```python
from build123d import *

# Parameters (mm, degrees)
SKETCH1_W                    = 80
SKETCH1_H                    = 40
SKETCH1_R                    = 10
BOSS_EXTRUDE1_DEPTH          = 3
SKETCH2_W                    = 80
SKETCH2_H                    = 4.5
BOSS_EXTRUDE2_DEPTH          = 8
SKETCH3_W                    = 2.5
SKETCH3_H                    = 6
CUT_EXTRUDE1_DEPTH           = 80
SKETCH5_R                    = 1.75
CUT_EXTRUDE3_DEPTH           = 1
SKETCH4_R                    = 3.75
CUT_EXTRUDE4_DEPTH           = 2
CUT_EXTRUDE4_DRAFT           = -45
CUT_EXTRUDE4_PROFILE_2_DEPTH = 2
CUT_EXTRUDE4_PROFILE_2_DRAFT = -45
CUT_EXTRUDE4_PROFILE_3_DEPTH = 2
CUT_EXTRUDE4_PROFILE_3_DRAFT = -45
CUT_EXTRUDE4_PROFILE_4_DEPTH = 2
CUT_EXTRUDE4_PROFILE_4_DRAFT = -45
FILLET1_R                    = 7
SKETCH6_W                    = 30
SKETCH6_H                    = 6
BOSS_EXTRUDE3_DEPTH          = 6
SKETCH7_R                    = 3
BOSS_EXTRUDE4_DEPTH          = 2


with BuildPart() as part:
    # Sketch1 → Boss-Extrude1 (new body)
    with BuildSketch(Plane(origin=(0, 0, 0), x_dir=(1, 0, 0), z_dir=(0, 1, 0))):
        Rectangle(SKETCH1_W, SKETCH1_H)
        with Locations(Location((0, 0, 0), (0, 0, 270))):
            Circle(SKETCH1_R, mode=Mode.SUBTRACT)
    extrude(amount=BOSS_EXTRUDE1_DEPTH)

    # Sketch2 → Boss-Extrude2 (add)
    with BuildSketch(Plane(origin=(0, 3, 0), x_dir=(1, 0, 0), z_dir=(0, 1, 0))):
        with Locations((0, 17.75)):
            Rectangle(SKETCH2_W, SKETCH2_H)
        with Locations((0, -17.75)):
            Rectangle(SKETCH2_W, SKETCH2_H)
    extrude(amount=BOSS_EXTRUDE2_DEPTH)

    # Sketch3 → Cut-Extrude1 (cut)
    with BuildSketch(Plane.ZY.offset(40)):
        with Locations((-16.75, 6)):
            Rectangle(SKETCH3_W, SKETCH3_H)
        with Locations((16.75, 6)):
            Rectangle(SKETCH3_W, SKETCH3_H)
    extrude(amount=-CUT_EXTRUDE1_DEPTH, mode=Mode.SUBTRACT)

    # Sketch5 → Cut-Extrude3 (cut)
    with BuildSketch(Plane.XZ):
        with Locations(Location((-15.5, 8, 0), (0, 0, 270))):
            Circle(SKETCH5_R)
        with Locations(Location((-15.5, -8, 0), (0, 0, 270))):
            Circle(SKETCH5_R)
        with Locations(Location((15.5, 8, 0), (0, 0, 270))):
            Circle(SKETCH5_R)
        with Locations(Location((15.5, -8, 0), (0, 0, 270))):
            Circle(SKETCH5_R)
    extrude(amount=-CUT_EXTRUDE3_DEPTH, mode=Mode.SUBTRACT)


with BuildPart() as cut_extrude4_tool:
    # Sketch4 → Cut-Extrude4 (with draft: the straight prism first)
    with BuildSketch(Plane(origin=(0, 3, 0), x_dir=(1, 0, 0), z_dir=(0, 1, 0))):
        with Locations((-15.5, 8)):
            Circle(SKETCH4_R)
    extrude(amount=-CUT_EXTRUDE4_DEPTH)
    # Cut-Extrude4: the draft: its side faces are tilted about the plane it starts from
    cut_extrude4_sides = [cut_extrude4_tool.faces().sort_by_distance(p)[0] for p in [
        (-19.25, 2, -8),
    ]]
    draft(cut_extrude4_sides, Plane(origin=(0, 3, 0), x_dir=(1, 0, 0), z_dir=(0, 1, 0)), CUT_EXTRUDE4_DRAFT)


with BuildPart() as part_1:
    add(part.part)

    # Cut-Extrude4: cut by cut_extrude4_tool
    add(cut_extrude4_tool.part, mode=Mode.SUBTRACT)


with BuildPart() as cut_extrude4_profile_2_tool:
    # Sketch4 → Cut-Extrude4 profile 2 (with draft: the straight prism first)
    with BuildSketch(Plane(origin=(0, 3, 0), x_dir=(1, 0, 0), z_dir=(0, 1, 0))):
        with Locations((-15.5, -8)):
            Circle(SKETCH4_R)
    extrude(amount=-CUT_EXTRUDE4_PROFILE_2_DEPTH)
    # Cut-Extrude4 profile 2: the draft: its side faces are tilted about the plane it starts from
    cut_extrude4_profile_2_sides = [cut_extrude4_profile_2_tool.faces().sort_by_distance(p)[0] for p in [
        (-19.25, 2, 8),
    ]]
    draft(cut_extrude4_profile_2_sides, Plane(origin=(0, 3, 0), x_dir=(1, 0, 0), z_dir=(0, 1, 0)), CUT_EXTRUDE4_PROFILE_2_DRAFT)


with BuildPart() as part_2:
    add(part_1.part)

    # Cut-Extrude4 profile 2: cut by cut_extrude4_profile_2_tool
    add(cut_extrude4_profile_2_tool.part, mode=Mode.SUBTRACT)


with BuildPart() as cut_extrude4_profile_3_tool:
    # Sketch4 → Cut-Extrude4 profile 3 (with draft: the straight prism first)
    with BuildSketch(Plane(origin=(0, 3, 0), x_dir=(1, 0, 0), z_dir=(0, 1, 0))):
        with Locations((15.5, -8)):
            Circle(SKETCH4_R)
    extrude(amount=-CUT_EXTRUDE4_PROFILE_3_DEPTH)
    # Cut-Extrude4 profile 3: the draft: its side faces are tilted about the plane it starts from
    cut_extrude4_profile_3_sides = [cut_extrude4_profile_3_tool.faces().sort_by_distance(p)[0] for p in [
        (11.75, 2, 8),
    ]]
    draft(cut_extrude4_profile_3_sides, Plane(origin=(0, 3, 0), x_dir=(1, 0, 0), z_dir=(0, 1, 0)), CUT_EXTRUDE4_PROFILE_3_DRAFT)


with BuildPart() as part_3:
    add(part_2.part)

    # Cut-Extrude4 profile 3: cut by cut_extrude4_profile_3_tool
    add(cut_extrude4_profile_3_tool.part, mode=Mode.SUBTRACT)


with BuildPart() as cut_extrude4_profile_4_tool:
    # Sketch4 → Cut-Extrude4 profile 4 (with draft: the straight prism first)
    with BuildSketch(Plane(origin=(0, 3, 0), x_dir=(1, 0, 0), z_dir=(0, 1, 0))):
        with Locations((15.5, 8)):
            Circle(SKETCH4_R)
    extrude(amount=-CUT_EXTRUDE4_PROFILE_4_DEPTH)
    # Cut-Extrude4 profile 4: the draft: its side faces are tilted about the plane it starts from
    cut_extrude4_profile_4_sides = [cut_extrude4_profile_4_tool.faces().sort_by_distance(p)[0] for p in [
        (11.75, 2, -8),
    ]]
    draft(cut_extrude4_profile_4_sides, Plane(origin=(0, 3, 0), x_dir=(1, 0, 0), z_dir=(0, 1, 0)), CUT_EXTRUDE4_PROFILE_4_DRAFT)


with BuildPart() as part_4:
    add(part_3.part)

    # Cut-Extrude4 profile 4: cut by cut_extrude4_profile_4_tool
    add(cut_extrude4_profile_4_tool.part, mode=Mode.SUBTRACT)

    # Fillet1
    fillet1_edges = [part_4.edges().sort_by_distance(p)[0] for p in [
        (40, 5.5, 20),
        (40, 5.5, -20),
        (-40, 5.5, 20),
        (-40, 5.5, -20),
    ]]
    fillet(fillet1_edges, radius=FILLET1_R)

    # Sketch6 → Boss-Extrude3 (add)
    with BuildSketch(Plane(origin=(0, 3, 0), x_dir=(1, 0, 0), z_dir=(0, 1, 0))):
        with Locations((-25, 0.145287111)):
            Rectangle(SKETCH6_W, SKETCH6_H)
        with Locations((25, 0.145287111)):
            Rectangle(SKETCH6_W, SKETCH6_H)
    extrude(amount=BOSS_EXTRUDE3_DEPTH)

    # Sketch7 → Boss-Extrude4 (add)
    with BuildSketch(Plane(origin=(0, 9, 0), x_dir=(1, 0, 0), z_dir=(0, 1, 0))):
        with BuildLine():
            Line((40, 6), (18.672144385, 6))
            ThreePointArc((18.672144385, 6), (15.5, 4.25), (12.327855615, 6))
            Line((12.327855615, 6), (-12.327855615, 6))
            ThreePointArc((-12.327855615, 6), (-15.5, 4.25), (-18.672144385, 6))
            Line((-18.672144385, 6), (-40, 6))
            Line((-40, 6), (-40, -6))
            Line((-40, -6), (-18.672144385, -6))
            ThreePointArc((-18.672144385, -6), (-15.5, -4.25), (-12.327855615, -6))
            Line((-12.327855615, -6), (12.327855615, -6))
            ThreePointArc((12.327855615, -6), (15.5, -4.25), (18.672144385, -6))
            Line((18.672144385, -6), (40, -6))
            Line((40, -6), (40, 6))
        make_face()
        with Locations(Location((0, 0, 0), (0, 0, 270))):
            Circle(SKETCH7_R, mode=Mode.SUBTRACT)
    extrude(amount=BOSS_EXTRUDE4_DEPTH)


solid = part_4.part
```
Input: part model. Units: mm. Frame: model coordinates. A direction names the side the tool comes from. Give positions to 0.01 mm unless a question says otherwise; leave off trailing zeros. Loops run counter-clockwise (first coordinate to the right, second up) from the corner with the lowest first, then second, coordinate; pieces in that order, holes last. Notation, with made-up numbers: M 57,49.25 L 79,49.25 A26 cw 79,72.25 Z; hole C 67.25,-39 d11. An arc over 180 degrees is marked long. Answer as CSV lines item,"result". Start each with the question number.
1. Line query: L1, parallel to X at y = 0.55, z = -8; L2, parallel to Z at x = -15.5, y = 0.3; L3, parallel to Z at x = -33.5, y = 6.5. Output: solid intervals per line, ascending.
2. Section A-A on x = 15.5. State how many separate pieces and enclosed holes the cut face has, plus the area to 3 significant figures.
3. Pull-direction query (Z, two-part tool) for faces 1 (the face through (0, 5, 20)), 2 (the face through (-10, 6, 0)), 3 (the face through (-1, 10, -15.5)), 4 (the face through (0, 5, -20)); classes: released by +Z, released by -Z, zero draft, split by the parting line, or undercut.
4. Pin query (flat end, axial travel): P1, Ø4.5, axis at x = 15.5, z = 8, coming from the +Y side; P2, Ø9.5, axis at x = -0.5, z = 1, coming from the -Y side. Return the tip coordinate at first contact, or that it passes through.
5. Section B-B on y = 7. Return loops of the section in (x, z), plus the area to 3 significant figures.
6. Section D-D on x = 0. Return loops of the section in (y, z).
7. Section C-C on z = 8. Return loops of the section in (x, y).
8. Reachability of faces 5 (the face through (-14, 0.5, -8.9)), 6 (the face through (29, 10, 6)), 7 (the face through (15.45, 9.99, 4.25)), 8 (the face through (36.95, 5.42, -18.78)), 9 (the face through (-1, 6, 18)) from +Z, -Z, +X, -X, +Y, -Y: full face, straight path, thin tool, end or side. Return the list, or none.
Computed values:
1,L1,"x = -40 to -17.25, -13.75 to -6, 6 to 13.75, 17.25 to 40"
1,L2,"z = -20 to -9.75, -6.25 to 6.25, 9.75 to 20"
1,L3,"z = -19.98 to -18, -3.15 to 2.85, 18 to 19.98"
2,separate pieces,"3"
2,enclosed holes,"0"
2,area,"186 mm²"
3,face 1,"released by +Z"
3,face 2,"undercut"
3,face 3,"undercut"
3,face 4,"released by -Z"
4,P1,"stops at y = 1.5"
4,P2,"stops at y = 9"
5,outline,"M -40,-3.15 L -10,-3.15 L -10,2.85 L -40,2.85 Z; M -37.9,-18 A7 ccw -33,-20 L 33,-20 A7 ccw 37.9,-18 Z; M -37.9,18 L 37.9,18 A7 ccw 33,20 L -33,20 A7 ccw Z; M 10,-3.15 L 40,-3.15 L 40,2.85 L 10,2.85 Z"
5,area,"651 mm²"
6,outline,"M 0,-20 L 11,-20 L 11,-15.5 L 9,-15.5 L 9,-18 L 3,-18 L 3,-10 L 0,-10 Z; M 0,10 L 3,10 L 3,18 L 9,18 L 9,15.5 L 11,15.5 L 11,20 L 0,20 Z; M 9,-6 L 11,-6 L 11,-3 L 9,-3 Z; M 9,3 L 11,3 L 11,6 L 9,6 Z"
7,outline,"M -40,0 L -17.25,0 L -17.25,1 L -19.25,3 L -40,3 Z; M -13.75,0 L -6,0 L -6,3 L -11.75,3 L -13.75,1 Z; M 6,0 L 13.75,0 L 13.75,1 L 11.75,3 L 6,3 Z; M 17.25,0 L 40,0 L 40,3 L 19.25,3 L 17.25,1 Z"
8,face 5,"+Y, -Y"
8,face 6,"+X, -X, +Y"
8,face 7,"+Y"
8,face 8,"-Z, +X, +Y, -Y"
8,face 9,"+X, -X"
